Model file for the job. Use its own axes, mm. A direction names the side the tool comes from. Round coordinates to 2 decimals unless told otherwise and drop trailing zeros. Loops run counter-clockwise (first coordinate to the right, second up) from the corner with the lowest first, then second, coordinate; pieces in that order, holes last. Notation, with made-up numbers: M 23,17 L 37,17 A12 cw 37,30 Z; hole C 40,26 d10. An arc over 180 degrees is marked long. Answer in a Markdown table with one row per item.
from build123d import *

# Parameters (mm, degrees)
SKETCH2_W               = 3
SKETCH2_H               = 0.5
CUT_EXTRUDE1_DEPTH      = 1.2
SKETCH3_R               = 0.2
BOSS_EXTRUDE1_DEPTH     = 17.5
SKETCH4_R               = 0.2
BOSS_EXTRUDE2_DEPTH     = 1.5
SKETCH5_W               = 5
SKETCH5_H               = 17
CUT_EXTRUDE2_DEPTH      = 2.9
CUT_EXTRUDE2_DEPTH_BACK = 2.9
SKETCH6_R               = 0.9
BOSS_EXTRUDE3_DEPTH     = 0.5
FILLET2_R               = 0.4
SKETCH7_R               = 0.6
BOSS_EXTRUDE4_DEPTH     = 1.6
FILLET3_R               = 0.1


with BuildPart() as part:
    # Sketch1 → Revolve1 (revolve)
    with BuildSketch(Plane.XY):
        with BuildLine():
            Line((0, 0), (0, 5.25))
            Line((0, 5.25), (0.1, 5.25))
            ThreePointArc((0.1, 5.25), (1.089949494, 4.839949494), (1.5, 3.85))
            Line((1.5, 3.85), (1.5, 1.2))
            Line((1.5, 1.2), (1.9, 1.2))
            Line((1.9, 1.2), (1.9, 0))
            Line((1.9, 0), (0, 0))
        make_face()
    revolve(axis=Axis((0, 0, 0), (0, 1, 0)))

    # Sketch2 → Cut-Extrude1 (cut)
    with BuildSketch(Plane(origin=(0, 1.2, 0), x_dir=(1, 0, 0), z_dir=(0, 1, 0))):
        with Locations((0, 1.78)):
            Rectangle(SKETCH2_W, SKETCH2_H)
    extrude(amount=-CUT_EXTRUDE1_DEPTH, mode=Mode.SUBTRACT)

    # Sketch3 → Boss-Extrude1 (add)
    with BuildSketch(Plane.XZ):
        with Locations((0, 1.27)):
            Circle(SKETCH3_R)
        with Locations((0, -1.27)):
            Circle(SKETCH3_R)
    extrude(amount=BOSS_EXTRUDE1_DEPTH)

    # Sketch4 → Boss-Extrude2 (add)
    with BuildSketch(Plane.XZ.offset(17.5)):
        with Locations((0, 1.27)):
            Circle(SKETCH4_R)
    extrude(amount=BOSS_EXTRUDE2_DEPTH)

    # Sketch5 → Cut-Extrude2 (cut, two sides)
    with BuildSketch(Plane(origin=(0, 0, 0), x_dir=(0, 0, -1), z_dir=(1, 0, 0))) as cut_extrude2_sk:
        with Locations((0, -10.5)):
            Rectangle(SKETCH5_W, SKETCH5_H)
    extrude(amount=CUT_EXTRUDE2_DEPTH, mode=Mode.SUBTRACT)
    extrude(cut_extrude2_sk.sketch, amount=-CUT_EXTRUDE2_DEPTH_BACK, mode=Mode.SUBTRACT)

    # Sketch6 → Boss-Extrude3 (add)
    with BuildSketch(Plane.XZ.offset(2)):
        with Locations((0, 1.27)):
            Circle(SKETCH6_R)
        with Locations((0, -1.27)):
            Circle(SKETCH6_R)
    extrude(amount=BOSS_EXTRUDE3_DEPTH)

    # Fillet2
    fillet2_edges = [part.edges().sort_by_distance(p)[0] for p in [
        (-0.9, -2.5, 1.27),
        (-0.9, -2.5, -1.27),
    ]]
    fillet(fillet2_edges, radius=FILLET2_R)

    # Sketch7 → Boss-Extrude4 (add)
    with BuildSketch(Plane(origin=(0, -2, 0), x_dir=(1, 0, 0), z_dir=(0, 1, 0))):
        with Locations((0, -1.27)):
            Circle(SKETCH7_R)
        with Locations((0, 1.27)):
            Circle(SKETCH7_R)
    extrude(amount=BOSS_EXTRUDE4_DEPTH)

    # Fillet3
    fillet3_edges = [part.edges().sort_by_distance(p)[0] for p in [
        (-0.6, -0.4, 1.27),
        (-0.6, -0.4, -1.27),
    ]]
    fillet(fillet3_edges, radius=FILLET3_R)


solid = part.part
1. Wall check: probe 1 along Y at (x, z) = (1.7, 0.1); probe 2 along Z at (x, y) = (0.35, 1); probe 3 along Z at (x, y) = (0.2, -0.75). Give the ranges that are in metal, low to high.
Verdict:
| item | result |
|---|---|
| probe 1 | y = 0 to 1.2 |
| probe 2 | z = -1.53 to 1.87 |
| probe 3 | z = -1.84 to -0.7, 0.7 to 1.84 |
2. Pin check, flat tips, straight feed: pin 1 (0.9 mm diameter, centred on x = 0.5, z = 1, fed in from +Y); pin 2 (1.5 mm diameter, centred on y = 0.5, z = -1.5, fed in from +X); pin 3 (0.9 mm diameter, centred on x = 0, z = -1.5, fed in from +Y). Stop position of each tip, or through.
Verdict:
| item | result |
|---|---|
| pin 1 | stops at y = 5.13 |
| pin 2 | stops at x = 1.75 |
| pin 3 | stops at y = 4.88 |
3. Tool access for faces 5 (the flat face through (0, -2.5, 1)), 6 (the flat face through (0, 1, -1.53)): list every direction of +Z, -Z, +X, -X, +Y, -Y with a clear straight run to the whole face (end or side of a thin tool).
Verdict:
| item | result |
|---|---|
| face 5 | +Z, -Z, +X, -X, -Y |
| face 6 | -Z, +X, -X, +Y |
4. Saw through at A-A (y = -1). Write the cut outline in (x, z), and give its area (3 significant figures).
Verdict:
| item | result |
|---|---|
| outline | C 0,-1.27 d1.2; C 0,1.27 d1.2 |
| area | 2.26 mm² |
5. Mould opens along Y. For faces 1 (the flat face through (0, -2.5, -1)), 2 (the cylindrical face through (0.323, -1.26, 0.764)), 3 (the cylindrical face through (-1.5, 2.51, -0.07)), 4 (the cylindrical face through (-0.13, -1.26, -0.684)) say: +Y half, -Y half, draft (parallel to the pull), parting line (faces both ways), or undercut.
Verdict:
| item | result |
|---|---|
| face 1 | -Y half |
| face 2 | undercut |
| face 3 | draft |
| face 4 | undercut |
